Can you work these out from the model? Positions are in its coordinate system, mm. A direction names the side the tool comes from. Give positions to 0.01 mm unless a question says otherwise; leave off trailing zeros. Write each loop counter-clockwise with the first axis right and the second up, starting at its lowest first coordinate (ties: lowest second). Pieces come first, ordered by that corner, then holes. Notation, with made-up numbers: (4, -13.75) -> (30, -13.75) arc R29 ccw to (30, 7.25) -> close; hole circle Ø5 at (-38.75, 80.5). An arc over 180 degrees is marked (long way). Answer as CSV lines item,"result". Start each with the question number.
1. On a 3-axis mill with a long thin cutter (end or side, diameter ignored), from which of +Z, -Z, +X, -X, +Y, -Y can I reach the whole of each face in a straight line? I mean faces 4 (the face through (-9.801, 5.056, 8.035)), 5 (the face through (-12, 5, 7.75)), 6 (the face through (16.64, 4.56, 14.1)). Say none if no direction works.
2. I need wall thicknesses on line 1 (Z direction, x = 13, y = 3.75); line 2 (X direction, y = 6.75, z = 11); line 3 (Z direction, x = 0, y = 0.6). Which ranges of each line are inside material? Lowest first, please. Write a range as [from, to].
3. If we section it at B-B on x = 0: Write out the boundary of the cut face in (y, z), plus the area to 3 significant figures.
4. I'm going to push a flat-ended pin straight in: P1, Ø3, axis at x = -13, z = -11, coming from the -Y side. Where does the tip first touch, or does it pass through?
5. If we section it at A-A on y = 6: Write out the boundary of the cut face in (x, z), plus the area to 3 significant figures.
6. If we section it at C-C on z = -11: Write out the boundary of the cut face in (x, y).
7. If we section it at D-D on x = 13: Write out the boundary of the cut face in (y, z), plus the area to 4 significant figures.
8. If we mould it in two halves opening along X, with no side actions, what happens to faces 1 (the face through (9.5, 5, -10)), 2 (the face through (-16.64, 4.56, 14.1)), 3 (the face through (17.5, 0.4, 0.2))? For each: pulls with the +X half, pulls with the -X half, needs draft (parallel to the pull), parting line crosses it, or undercut.
```python
from build123d import *

# Parameters (mm, degrees)
SKETCH1_W            = 35
SKETCH1_H            = 30
BOSS_EXTRUDE1_DEPTH  = 9
SKETCH3_W            = 29
SKETCH3_H            = 24
CUT_EXTRUDE1_DEPTH   = 8
SKETCH4_W            = 15.5
SKETCH4_H            = 8.1
CUT_EXTRUDE2_DEPTH   = 36
SKETCH5_W            = 5
SKETCH5_H            = 4.25
BOSS_EXTRUDE2_DEPTH  = 8
M3_CLEARANCE_HOLE1_D = 3.6
FILLET1_R            = 3
FILLET2_R            = 1


with BuildPart() as part:
    # Sketch1 → Boss-Extrude1 (new body)
    with BuildSketch(Plane(origin=(0, 0, 0), x_dir=(1, 0, 0), z_dir=(0, 1, 0))):
        Rectangle(SKETCH1_W, SKETCH1_H)
    extrude(amount=BOSS_EXTRUDE1_DEPTH)

    # Sketch3 → Cut-Extrude1 (cut)
    with BuildSketch(Plane(origin=(0, 9, 0), x_dir=(1, 0, 0), z_dir=(0, 1, 0))):
        Rectangle(SKETCH3_W, SKETCH3_H)
    extrude(amount=-CUT_EXTRUDE1_DEPTH, mode=Mode.SUBTRACT)

    # Sketch4 → Cut-Extrude2 (cut, through all)
    with BuildSketch(Plane.ZY.offset(17.5)):
        with Locations((0, 4.95)):
            Rectangle(SKETCH4_W, SKETCH4_H)
    extrude(amount=-CUT_EXTRUDE2_DEPTH, mode=Mode.SUBTRACT)

    # Sketch5 → Boss-Extrude2 (add)
    with BuildSketch(Plane(origin=(0, 1, 0), x_dir=(1, 0, 0), z_dir=(0, 1, 0))):
        with Locations((-12, 9.875)):
            Rectangle(SKETCH5_W, SKETCH5_H)
        with Locations((12, 9.875)):
            Rectangle(SKETCH5_W, SKETCH5_H)
        with Locations((12, -9.875)):
            Rectangle(SKETCH5_W, SKETCH5_H)
        with Locations((-12, -9.875)):
            Rectangle(SKETCH5_W, SKETCH5_H)
    extrude(amount=BOSS_EXTRUDE2_DEPTH)

    # M3 Clearance Hole1 (through all)
    with Locations(Plane(origin=(0, 9, 0), x_dir=(1, 0, 0), z_dir=(0, 1, 0))):
        with Locations((0, 0), (13, 11), (-13, -11), (-13, 11), (13, -11)):
            Hole(M3_CLEARANCE_HOLE1_D / 2)

    # Fillet1
    fillet1_edges = [part.edges().sort_by_distance(p)[0] for p in [
        (17.5, 4.5, 15),
        (-17.5, 4.5, 15),
        (-17.5, 4.5, -15),
        (17.5, 4.5, -15),
    ]]
    fillet(fillet1_edges, radius=FILLET1_R)

    # Fillet2
    fillet2_edges = [part.edges().sort_by_distance(p)[0] for p in [
        (-9.5, 5, -7.75),
        (9.5, 5, -7.75),
        (9.5, 5, 7.75),
        (-9.5, 5, 7.75),
    ]]
    fillet(fillet2_edges, radius=FILLET2_R)


solid = part.part
```
Computed values:
1,face 4,"+Y"
1,face 5,"+X, -X, +Y"
1,face 6,"+Z, +X, +Y, -Y"
2,line 1,"z = [-15, -12.8], [-9.2, -7.75], [7.75, 9.2], [12.8, 15]"
2,line 2,"x = [-17.5, -14.8], [-11.2, -9.5], [9.5, 11.2], [14.8, 17.5]"
2,line 3,"z = [-15, -1.8], [1.8, 15]"
3,outline,"(0, -15) -> (9, -15) -> (9, -12) -> (1, -12) -> (1, -7.75) -> (0.9, -7.75) -> (0.9, -1.8) -> (0, -1.8) -> close; (0, 1.8) -> (0.9, 1.8) -> (0.9, 7.75) -> (1, 7.75) -> (1, 12) -> (9, 12) -> (9, 15) -> (0, 15) -> close"
3,area,"73.2 mm2"
4,P1,"passes through"
5,outline,"(-17.5, -12) arc R3 ccw to (-14.5, -15) -> (14.5, -15) arc R3 ccw to (17.5, -12) -> (17.5, -7.75) -> (10.5, -7.75) arc R1 ccw to (9.5, -8.75) -> (9.5, -12) -> (-9.5, -12) -> (-9.5, -8.75) arc R1 ccw to (-10.5, -7.75) -> (-17.5, -7.75) -> close; (-17.5, 7.75) -> (-10.5, 7.75) arc R1 ccw to (-9.5, 8.75) -> (-9.5, 12) -> (9.5, 12) -> (9.5, 8.75) arc R1 ccw to (10.5, 7.75) -> (17.5, 7.75) -> (17.5, 12) arc R3 ccw to (14.5, 15) -> (-14.5, 15) arc R3 ccw to (-17.5, 12) -> close; hole circle Ø3.6 at (-13, -11); hole circle Ø3.6 at (-13, 11); hole circle Ø3.6 at (13, -11); hole circle Ø3.6 at (13, 11)"
5,area,"297 mm2"
6,outline,"(-17.5, 0) -> (-14.8, 0) -> (-14.8, 9) -> (-17.5, 9) -> close; (-11.2, 0) -> (11.2, 0) -> (11.2, 9) -> (9.5, 9) -> (9.5, 1) -> (-9.5, 1) -> (-9.5, 9) -> (-11.2, 9) -> close; (14.8, 0) -> (17.5, 0) -> (17.5, 9) -> (14.8, 9) -> close"
7,outline,"(0, -15) -> (9, -15) -> (9, -12.8) -> (0, -12.8) -> close; (0, -9.2) -> (9, -9.2) -> (9, -7.75) -> (0.9, -7.75) -> (0.9, 7.75) -> (9, 7.75) -> (9, 9.2) -> (0, 9.2) -> close; (0, 12.8) -> (9, 12.8) -> (9, 15) -> (0, 15) -> close"
7,area,"79.65 mm2"
8,face 1,"undercut"
8,face 2,"pulls with the -X half"
8,face 3,"pulls with the +X half"
